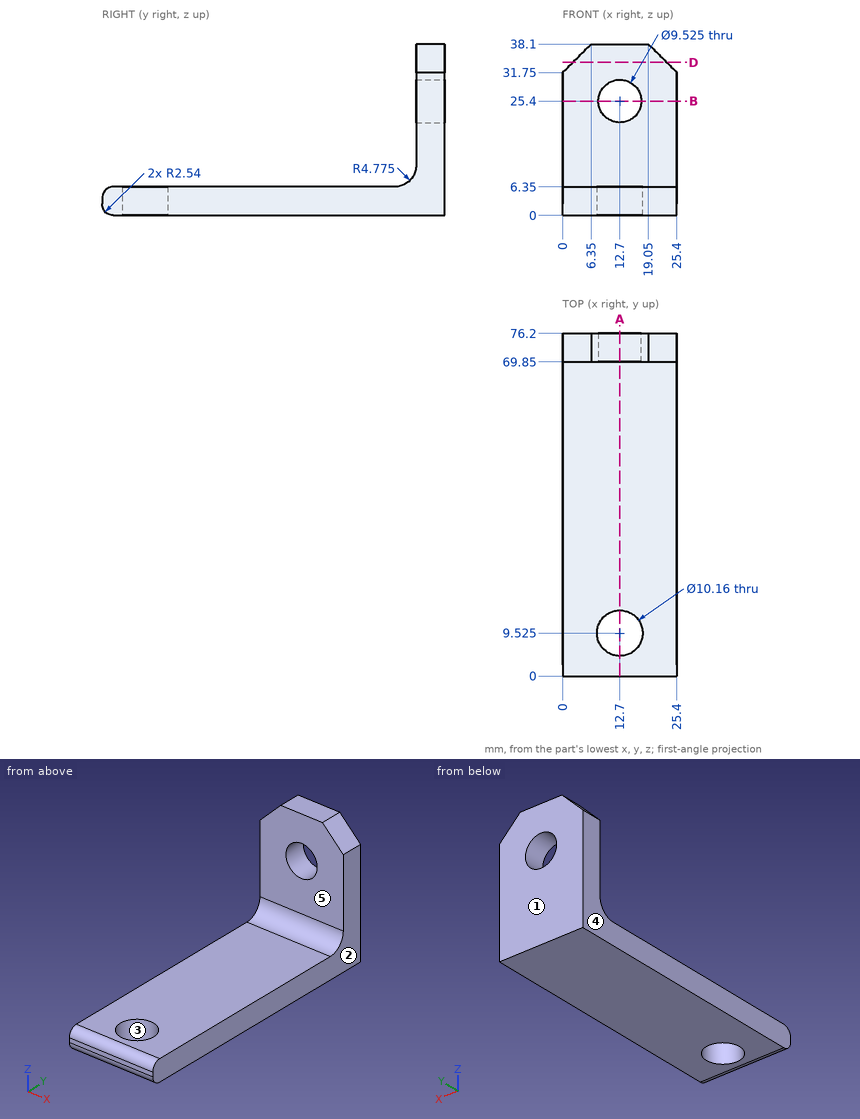
Study the drawing (mm; zero at the part's minimum x, y, z) and answer. A direction names the side the tool comes from. Round coordinates to 2 decimals unless told otherwise and drop trailing zeros. Write each loop counter-clockwise with the first axis right and the second up, starting at its lowest first coordinate (ties: lowest second). Pieces come first, ordered by that corner, then holes. Notation, with made-up numbers: (27.25, 68) - (57.25, 68) arc R16 ccw to (57.25, 87) - close; hole circle Ø8 at (0.5, 9). An arc over 180 degrees is marked (long way). Return JSON: item names as keys, results as strings. Group by question number.
Q1. For the marked faces 4 and 5, determine the directions among +Z, -Z, +X, -X, +Y, -Y from which every point of the face is accessible in a straight line to the end or side of a thin tool.
Q2. Each of these flat-tipped pins is pushed along its axis until it touches: pin 1 Ø8 at (x, y) = (7.5, 60) entering from +Z; pin 2 Ø12 at (x, z) = (12, 34) entering from -Y. Where does it stop, or does it pass through?
Q3. Find the intervals of material crossed by L1, parallel to Z at x = 12.7, y = 73.75; L2, parallel to Y at x = 8.75, z = 28.5; L3, parallel to Z at x = 8.5, y = 57, in increasing order.
Q4. The part is cut by section B-B on z = 25.4. Write down the section's boundary in (x, y).
Q5. The mould has two halves that part along Y. Classify the marked faces 1, 2 and 3: released by +Y, released by -Y, zero draft, split by the parting line, or undercut.
Q6. The part is cut by section D-D on z = 34. Write down the section's boundary in (x, y).
Q7. The part is cut by section A-A on x = 12.7. Count the separate pieces of the cut face and the enclosed holes in it, then the cut area to 3 significant figures.
Solved:
{
 "1": {"face 4": "+Z, -Z, -X, +Y, -Y", "face 5": "+Z, +X, -X, -Y"},
 "2": {"pin 1": "z = 6.35", "pin 2": "y = 69.85"},
 "3": {"L1": "0 to 20.64, 30.16 to 38.1", "L2": "69.85 to 76.2", "L3": "0 to 6.35"},
 "4": {"outline": "(0, 69.85) - (7.94, 69.85) - (7.94, 76.2) - (0, 76.2) - close; (17.46, 69.85) - (25.4, 69.85) - (25.4, 76.2) - (17.46, 76.2) - close"},
 "5": {"face 1": "released by +Y", "face 2": "zero draft", "face 3": "undercut"},
 "6": {"outline": "(2.25, 69.85) - (23.15, 69.85) - (23.15, 76.2) - (2.25, 76.2) - close"},
 "7": {"separate pieces": "3", "enclosed holes": "0", "area": "563 mm²"}
}
